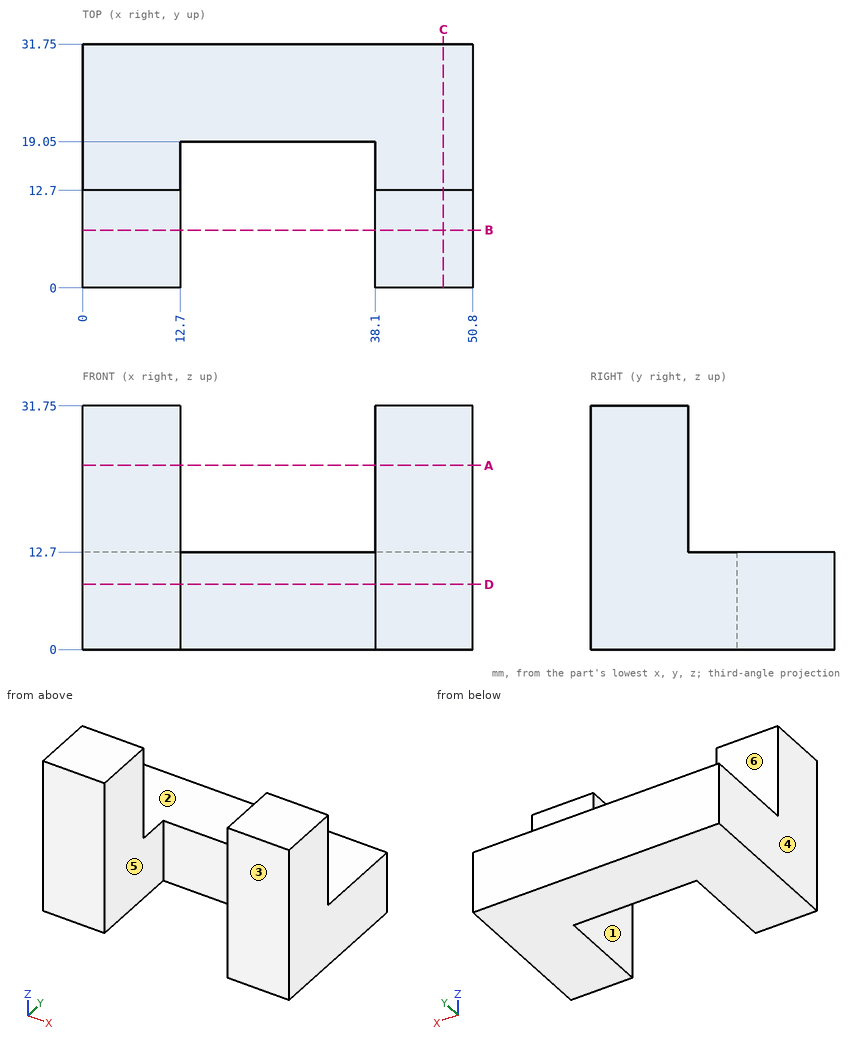
Input: dimensioned drawing with shaded views. Units: mm. Origin: part minimum x, y, z. A direction names the side the tool comes from. Give positions to 0.01 mm unless a question says otherwise; leave off trailing zeros. Order: outer loops, then holes, each group sorted by start corner. A loop starts at its lowest first (then second) coordinate and runs counter-clockwise, first axis right, second up.
(1) Pull-direction query (X, two-part tool) for the marked faces 4, 5 and 6; classes: +X half, -X half, draft (parallel to the pull), parting line (faces both ways), or undercut.
(2) Contact query for flat-ended pins moving along their axis: P1, Ø6.5, axis at x = 42, z = 21, coming from the +Y side; P2, Ø1.5, axis at x = 20, z = 10, coming from the -Y side; P3, Ø4, axis at x = 29.5, y = 23, coming from the +Z side. Output: stop coordinate, or through.
(3) Access query for the marked faces 1, 2 and 3. Directions: +Z, -Z, +X, -X, +Y, -Y. A direction counts if a zero-diameter tool reaches every point of the face in a straight line with its end or side. Return the directions, or none.
(4) Material intervals for line 1 along X through (y, z) = (3.5, 9.5); line 2 along Y through (x, z) = (44.5, 14.5), sorted ascending.
(5) Section query C-C (x = 47). Return the cut outline in (y, z).
(6) Section query D-D (z = 8.5). Return the cut outline in (x, y), plus the area to 3 significant figures.
(7) Section query B-B (y = 7.5). Return the cut outline in (x, z), plus the area to 3 significant figures.
(8) Section query A-A (z = 24). Return the cut outline in (x, y), plus the area to 3 significant figures.
Outcome:
1. face 4: -X half
1. face 5: undercut
1. face 6: draft
2. P1: stops at y = 12.7
2. P2: stops at y = 19.05
2. P3: stops at z = 12.7
3. face 1: +Z, -Z, -Y
3. face 2: +Z, +X, -X, +Y
3. face 3: +Z, -Z, +X, -X, -Y
4. line 1: x = 0 to 12.7, 38.1 to 50.8
4. line 2: y = 0 to 12.7
5. outline: (0, 0) - (31.75, 0) - (31.75, 12.7) - (12.7, 12.7) - (12.7, 31.75) - (0, 31.75) - close
6. outline: (0, 0) - (12.7, 0) - (12.7, 19.05) - (38.1, 19.05) - (38.1, 0) - (50.8, 0) - (50.8, 31.75) - (0, 31.75) - close
6. area: 1,130 mm2
7. outline: (0, 0) - (12.7, 0) - (12.7, 31.75) - (0, 31.75) - close; (38.1, 0) - (50.8, 0) - (50.8, 31.75) - (38.1, 31.75) - close
7. area: 806 mm2
8. outline: (0, 0) - (12.7, 0) - (12.7, 12.7) - (0, 12.7) - close; (38.1, 0) - (50.8, 0) - (50.8, 12.7) - (38.1, 12.7) - close
8. area: 323 mm2
